Design review of the part shown in the three views and the two pictorial views. Dimensions are in mm from the part's minimum x, y and z. Coordinates: 2 decimals unless noted, no trailing zeros. Write each loop counter-clockwise with the first axis right and the second up, starting at its lowest first coordinate (ties: lowest second). Pieces come first, ordered by that corner, then holes.
Q1. For pin 1 Ø2 at (y, z) = (1.5, 90) entering from +X; pin 2 Ø2 at (x, y) = (69, 1.5) entering from +Z; pin 3 Ø1.5 at (y, z) = (1, 11.5) entering from +X (1 decimal), all flat-tipped, find the tip position at first contact; note any pin that passes through.
Q2. Take a section at B-B, the plane x = 13. Write out the cut boundary in (y, z) (1 decimal).
Q3. Take a section at D-D, the plane z = 31. Write out the cut boundary in (x, y).
Q4. For L1, parallel to Z at x = 54.5, y = 1.1; L2, parallel to Z at x = 95, y = 4.05 (1 decimal); L3, parallel to Z at x = 7.5, y = 1.1 (1 decimal), list the stretches that pass through material, from the lowest coordinate up.
Q5. Take a section at C-C, the plane x = 57. Write out the cut boundary in (y, z), plus the area to 3 significant figures.
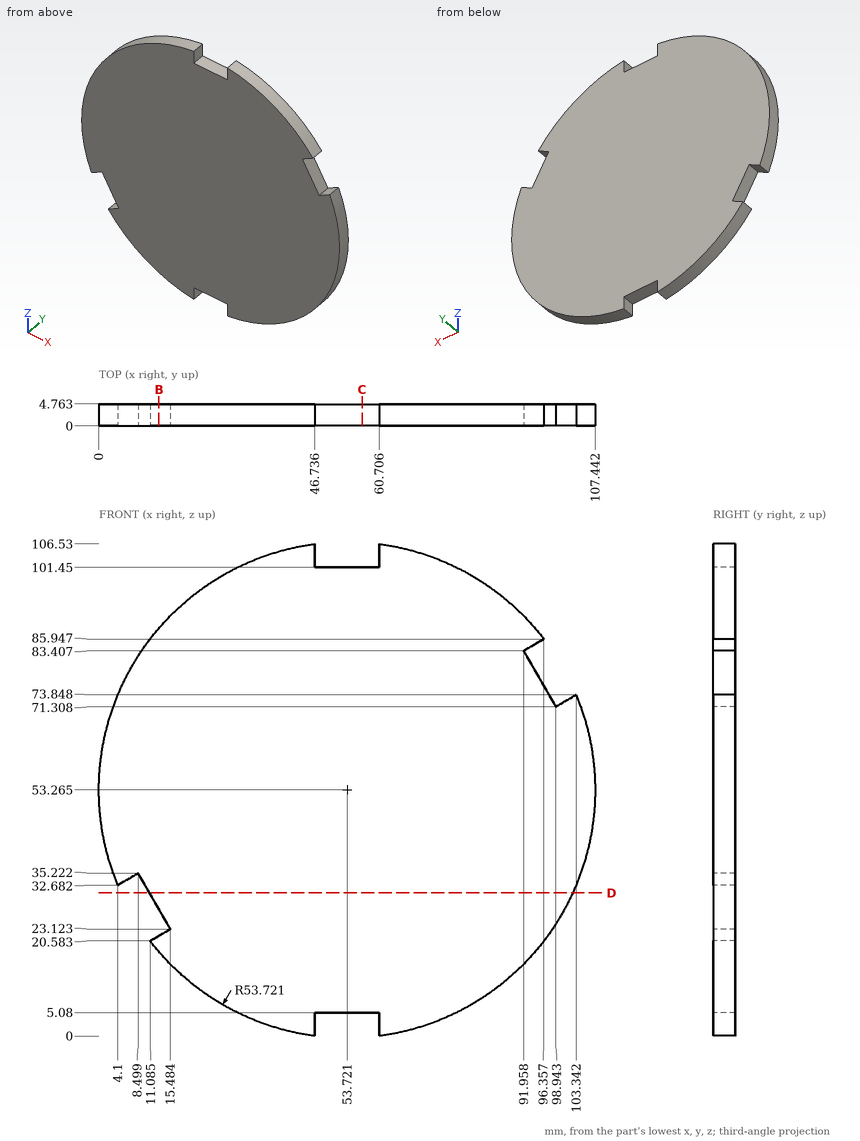
Responses:
1. pin 1: stops at x = 93.83
1. pin 2: stops at z = 105.05
1. pin 3: stops at x = 88.4
2. outline: (0, 18.2) - (4.8, 18.2) - (4.8, 21.7) - (0, 21.7) - close; (0, 27.4) - (4.8, 27.4) - (4.8, 88.3) - (0, 88.3) - close
3. outline: (10.94, 0) - (102.61, 0) - (102.61, 4.76) - (10.94, 4.76) - close
4. L1: z = 5.08 to 101.45
4. L2: z = 18.9 to 78.1, 85.2 to 87.6
4. L3: z = 34.6 to 80.6
5. outline: (0, 5.08) - (4.76, 5.08) - (4.76, 101.45) - (0, 101.45) - close
5. area: 459 mm2
